Geometry check sheet. Reference: the model listing, model coordinates, mm. A direction names the side the tool comes from. Coordinates: 2 decimals unless noted, no trailing zeros. Order: outer loops, then holes, each group sorted by start corner. A loop starts at its lowest first (then second) coordinate and runs counter-clockwise, first axis right, second up. Notation, with made-up numbers: (13.5, -11.5) -> (50.5, -11.5) arc R26 cw to (50.5, 18.5) -> close; hole circle Ø2 at (62, -9.75). An arc over 180 degrees is marked (long way). Answer as CSV lines item,"result". Start each with the question number.
from build123d import *

# Parameters (mm, degrees)
SLIDER_MAIN_BODY_DEPTH = 5
SKETCH2_W              = 1.666666666
SKETCH2_H              = 5
TRACK_SLIDER_DEPTH     = 1.666666667
SKETCH3_W              = 5
SKETCH3_H              = 15
HANDLE_DEPTH           = 5
SKETCH4_W              = 105
SKETCH4_H              = 1.666666666
CUT_EXTRUDE1_DEPTH     = 66.954529791
SKETCH5_W              = 1.666666667
SKETCH5_H              = 5
CUT_EXTRUDE2_DEPTH     = 5


with BuildPart() as part:
    # Sketch1 → Slider Main Body (new body)
    with BuildSketch(Plane.XY):
        Polygon((-55, 7.5), (-55, 2.5), (55, 2.5), (55, 7.5), (60, 7.5), (60, -7.5), (55, -7.5), (55, -2.5), (-55, -2.5), (-55, -7.5), (-60, -7.5), (-60, 7.5), align=None)
    extrude(amount=SLIDER_MAIN_BODY_DEPTH)

    # Sketch2 → Track Slider (add)
    with BuildSketch(Plane.XZ.offset(7.5)):
        with Locations((-57.5, 2.5)):
            Rectangle(SKETCH2_W, SKETCH2_H)
    extrude(amount=TRACK_SLIDER_DEPTH)

    # Sketch3 → Handle (add)
    with BuildSketch(Plane.XY.offset(5)):
        with Locations((-62.5, 0)):
            Rectangle(SKETCH3_W, SKETCH3_H)
    extrude(amount=-HANDLE_DEPTH)

    # Sketch4 → Cut-Extrude1 (cut, through all)
    with BuildSketch(Plane.XZ.offset(2.5)):
        with Locations((-2.5, 2.5)):
            Rectangle(SKETCH4_W, SKETCH4_H)
    extrude(amount=-CUT_EXTRUDE1_DEPTH, mode=Mode.SUBTRACT)

    # Sketch5 → Cut-Extrude2 (cut)
    with BuildSketch(Plane(origin=(0, 7.5, 0), x_dir=(1, 0, 0), z_dir=(0, 1, 0))):
        with Locations((-55.833333334, -2.5)):
            Rectangle(SKETCH5_W, SKETCH5_H)
    extrude(amount=-CUT_EXTRUDE2_DEPTH, mode=Mode.SUBTRACT)


solid = part.part
Q1. Go/stop test with flat-tipped pins: pin 1 Ø1.3 at (x, z) = (-55.5, 3.5) entering from -Y; pin 2 Ø1.5 at (x, z) = (-13.5, 3) entering from +Y; pin 3 Ø0.8 at (y, z) = (-8.5, 3.5) entering from -X; pin 4 Ø1 at (x, y) = (44, -4) entering from +Z. Record where each tip stops, or that it passes through.
Q2. Access from +Z, -Z, +X, -X, +Y, -Y to the whole of each face (thin tool, end or side, straight path). Record for faces 4 (the flat face through (-3, 0, 1.667)), 5 (the flat face through (1, -2.5, 1)), 6 (the flat face through (55, 5, 2)).
Q3. Sectioned sample at C-C, the plane z = 4.1. Record the cut outline in (x, y), then the cut area to 3 significant figures.
Q4. Release check for a two-part mould opening along X. For faces 1 (the flat face through (-3, 0, 3.333)), 2 (the flat face through (-7, 0, 0)), 3 (the flat face through (-65, 0, 3)) record: released by +X, released by -X, zero draft, split by the parting line, or undercut.
Q5. Sectioned sample at A-A, the plane y = 5.25. Record the cut outline in (x, z).
Q6. Thickness scan on L1, parallel to X at y = 6, z = 0.25; L2, parallel to Z at x = 28, y = 0.5; L3, parallel to X at y = -0.5, z = 2.9. Record the ranges inside material, lowest first.
Q7. Sectioned sample at B-B, the plane x = -7.5. Record the cut outline in (y, z), then the cut area to 3 significant figures.
Geometry results:
1,pin 1,"stops at y = -7.5"
1,pin 2,"stops at y = 2.5"
1,pin 3,"stops at x = -58.33"
1,pin 4,"passes through"
2,face 4,"+Y, -Y"
2,face 5,"+Z, -Z, -Y"
2,face 6,"+Z, -Z, +Y"
3,outline,"(-65, -7.5) -> (-58.33, -7.5) -> (-58.33, -9.17) -> (-56.67, -9.17) -> (-56.67, -7.5) -> (-55, -7.5) -> (-55, -2.5) -> (55, -2.5) -> (55, -7.5) -> (60, -7.5) -> (60, 7.5) -> (55, 7.5) -> (55, 2.5) -> (-56.67, 2.5) -> (-56.67, 7.5) -> (-65, 7.5) -> close"
3,area,"769 mm^2"
4,face 1,"undercut"
4,face 2,"zero draft"
4,face 3,"released by -X"
5,outline,"(-65, 0) -> (-56.67, 0) -> (-56.67, 5) -> (-65, 5) -> close; (55, 0) -> (60, 0) -> (60, 5) -> (55, 5) -> close"
6,L1,"x = -65 to -56.67, 55 to 60"
6,L2,"z = 0 to 1.67, 3.33 to 5"
6,L3,"x = -65 to -55, 50 to 60"
7,outline,"(-2.5, 0) -> (2.5, 0) -> (2.5, 1.67) -> (-2.5, 1.67) -> close; (-2.5, 3.33) -> (2.5, 3.33) -> (2.5, 5) -> (-2.5, 5) -> close"
7,area,"16.7 mm^2"
